Input: part model. Units: mm. Frame: model coordinates. A direction names the side the tool comes from. Give positions to 0.01 mm unless a question says otherwise; leave off trailing zeros. Loops run counter-clockwise (first coordinate to the right, second up) from the corner with the lowest first, then second, coordinate; pieces in that order, holes last. Notation, with made-up numbers: (54.5, 78.5) - (96.5, 78.5) arc R21 cw to (96.5, 106.5) - close; hole circle Ø3 at (69.25, 82.5). An arc over 180 degrees is marked (long way). Answer as a JSON object with one key per item and string values.
from build123d import *

# Parameters (mm, degrees)
BOSS_EXTRUDE1_DEPTH  = 9.2
FILLET1_R            = 0.3
CUT_EXTRUDE1_DEPTH   = 19.2
SKETCH3_W            = 9.9
SKETCH3_H            = 1.3
BOSS_EXTRUDE2_DEPTH  = 6.5
SKETCH4_W            = 0.621842352
SKETCH4_H            = 1.7
CUT_EXTRUDE3_DEPTH   = 16.5
SKETCH5_R            = 1.8
CUT_EXTRUDE4_DEPTH   = 16.5
SKETCH8_W            = 1.27
SKETCH8_H            = 0.5
BOSS_EXTRUDE4_DEPTH  = 1.46
SKETCH9_W            = 1.52
SKETCH9_H            = 0.5
BOSS_EXTRUDE5_DEPTH  = 1
SKETCH10_W           = 1.27
SKETCH10_H           = 0.5
BOSS_EXTRUDE6_DEPTH  = 0.5
SKETCH11_W           = 0.8
SKETCH11_H           = 0.5
BOSS_EXTRUDE7_DEPTH  = 10.08
CHAMFER1_SIZE        = 0.3
CHAMFER2_SIZE        = 0.2
BOSS_EXTRUDE10_DEPTH = 0.05


with BuildPart() as part:
    # Sketch1 → Boss-Extrude1 (new body)
    with BuildSketch(Plane.XY):
        Polygon((1.031077827, 0), (-8.968922173, 0), (-8.575223187, 4.5), (0.637378841, 4.5), align=None)
    extrude(amount=BOSS_EXTRUDE1_DEPTH)

    # Fillet1
    fillet1_edges = [part.edges().sort_by_distance(p)[0] for p in [
        (-8.575223187, 4.5, 4.6),
        (0.637378841, 4.5, 4.6),
    ]]
    fillet(fillet1_edges, radius=FILLET1_R)

    # Sketch2 → Cut-Extrude1 (cut)
    with BuildSketch(Plane(origin=(5, 0, 0), x_dir=(0, 0, -1), z_dir=(1, 0, 0))):
        Polygon((0, 4.5), (-0.279963723, 4.5), (0, 1.3), align=None)
    extrude(amount=-CUT_EXTRUDE1_DEPTH, mode=Mode.SUBTRACT)

    # Sketch3 → Boss-Extrude2 (add)
    with BuildSketch(Plane(origin=(0, 0, 0), x_dir=(-1, 0, 0), z_dir=(0, 0, -1))):
        with Locations((3.968922173, 0.65)):
            Rectangle(SKETCH3_W, SKETCH3_H)
    extrude(amount=BOSS_EXTRUDE2_DEPTH)

    # Sketch4 → Cut-Extrude3 (cut)
    with BuildSketch(Plane(origin=(0, 1.3, 0), x_dir=(1, 0, 0), z_dir=(0, 1, 0))):
        with Locations((-8.608000997, 4.35)):
            Rectangle(SKETCH4_W, SKETCH4_H)
        with Locations((0.670156651, 4.35)):
            Rectangle(SKETCH4_W, SKETCH4_H)
    extrude(amount=-CUT_EXTRUDE3_DEPTH, mode=Mode.SUBTRACT)

    # Sketch5 → Cut-Extrude4 (cut)
    with BuildSketch(Plane(origin=(0, 1.3, 0), x_dir=(1, 0, 0), z_dir=(0, 1, 0))):
        with Locations(Location((-3.968922173, 3.7, 0), (0, 0, 270))):
            Circle(SKETCH5_R)
    extrude(amount=-CUT_EXTRUDE4_DEPTH, mode=Mode.SUBTRACT)

    # Sketch8 → Boss-Extrude4 (add)
    with BuildSketch(Plane.XY.offset(9.2)):
        with Locations((-1.428922173, 2.4)):
            Rectangle(SKETCH8_W, SKETCH8_H)
        with Locations((-3.968922173, 2.4)):
            Rectangle(SKETCH8_W, SKETCH8_H)
        with Locations((-6.508922173, 2.4)):
            Rectangle(SKETCH8_W, SKETCH8_H)
    extrude(amount=BOSS_EXTRUDE4_DEPTH)

    # Sketch9 → Boss-Extrude5 (add)
    with BuildSketch(Plane.XY.offset(10.66)):
        with Locations((-3.968922173, 2.4)):
            Rectangle(SKETCH9_W, SKETCH9_H)
        with Locations((-1.428922173, 2.4)):
            Rectangle(SKETCH9_W, SKETCH9_H)
        with Locations((-6.508922173, 2.4)):
            Rectangle(SKETCH9_W, SKETCH9_H)
    extrude(amount=BOSS_EXTRUDE5_DEPTH)

    # Sketch10 → Boss-Extrude6 (add)
    with BuildSketch(Plane.XY.offset(11.66)):
        with Locations((-3.968922173, 2.4)):
            Rectangle(SKETCH10_W, SKETCH10_H)
        with Locations((-1.428922173, 2.4)):
            Rectangle(SKETCH10_W, SKETCH10_H)
        with Locations((-6.508922173, 2.4)):
            Rectangle(SKETCH10_W, SKETCH10_H)
    extrude(amount=BOSS_EXTRUDE6_DEPTH)

    # Sketch11 → Boss-Extrude7 (add)
    with BuildSketch(Plane.XY.offset(12.16)):
        with Locations((-3.968922173, 2.4)):
            Rectangle(SKETCH11_W, SKETCH11_H)
        with Locations((-1.428922173, 2.4)):
            Rectangle(SKETCH11_W, SKETCH11_H)
        with Locations((-6.508922173, 2.4)):
            Rectangle(SKETCH11_W, SKETCH11_H)
    extrude(amount=BOSS_EXTRUDE7_DEPTH)

    # Chamfer1
    # the kernel refuses this chamfer: 0.3 mm, written as the material it takes off along each edge
    with BuildSketch(Plane(origin=(-0.793922173, 3.421504896, 12.16), x_dir=(-0.9996219169112968, 0, 0.027495876610584464), z_dir=(0, -1, 0))) as chamfer1_piece_1_section:
        Polygon((CHAMFER1_SIZE * 0.999621916911, CHAMFER1_SIZE * 0.0274958766106), (-CHAMFER1_SIZE * 0.0274958766106, CHAMFER1_SIZE * 0.999621916911), (0, 0), align=None)
    chamfer1_piece_1 = extrude(amount=2.043009793, mode=Mode.PRIVATE)
    chamfer1_piece_1 = split(chamfer1_piece_1, bisect_by=Plane(origin=(-1.028922173, 2.4, 12.055687512), z_dir=(1, 0, 0)), keep=Keep.TOP, mode=Mode.PRIVATE)
    add(chamfer1_piece_1, mode=Mode.SUBTRACT)
    with BuildSketch(Plane(origin=(-2.063922173, 1.378495104, 12.16), x_dir=(-0.027495876610585904, 0, -0.9996219169112968), z_dir=(0, 1, 0))) as chamfer1_piece_2_section:
        Polygon((CHAMFER1_SIZE * 0.999621916911, -CHAMFER1_SIZE * 0.0274958766106), (-CHAMFER1_SIZE * 0.0274958766106, -CHAMFER1_SIZE * 0.999621916911), (0, 0), align=None)
    chamfer1_piece_2 = extrude(amount=2.043009793, mode=Mode.PRIVATE)
    chamfer1_piece_2 = split(chamfer1_piece_2, bisect_by=Plane(origin=(-1.828922173, 2.4, 12.055687512), z_dir=(-1, 0, 0)), keep=Keep.TOP, mode=Mode.PRIVATE)
    add(chamfer1_piece_2, mode=Mode.SUBTRACT)
    with BuildSketch(Plane(origin=(-4.603922173, 1.378495104, 12.16), x_dir=(-0.027495876610587344, 0, -0.9996219169112968), z_dir=(0, 1, 0))) as chamfer1_piece_3_section:
        Polygon((CHAMFER1_SIZE * 0.999621916911, -CHAMFER1_SIZE * 0.0274958766106), (-CHAMFER1_SIZE * 0.0274958766106, -CHAMFER1_SIZE * 0.999621916911), (0, 0), align=None)
    chamfer1_piece_3 = extrude(amount=2.043009793, mode=Mode.PRIVATE)
    chamfer1_piece_3 = split(chamfer1_piece_3, bisect_by=Plane(origin=(-4.368922173, 2.4, 12.055687512), z_dir=(-1, 0, 0)), keep=Keep.TOP, mode=Mode.PRIVATE)
    add(chamfer1_piece_3, mode=Mode.SUBTRACT)
    with BuildSketch(Plane(origin=(-3.333922173, 3.421504896, 12.16), x_dir=(-0.9996219169112968, 0, 0.027495876610584506), z_dir=(0, -1, 0))) as chamfer1_piece_4_section:
        Polygon((CHAMFER1_SIZE * 0.999621916911, CHAMFER1_SIZE * 0.0274958766106), (-CHAMFER1_SIZE * 0.0274958766106, CHAMFER1_SIZE * 0.999621916911), (0, 0), align=None)
    chamfer1_piece_4 = extrude(amount=2.043009793, mode=Mode.PRIVATE)
    chamfer1_piece_4 = split(chamfer1_piece_4, bisect_by=Plane(origin=(-3.568922173, 2.4, 12.055687512), z_dir=(1, 0, 0)), keep=Keep.TOP, mode=Mode.PRIVATE)
    add(chamfer1_piece_4, mode=Mode.SUBTRACT)
    with BuildSketch(Plane(origin=(-7.143922173, 1.378495104, 12.16), x_dir=(-0.027495876610587344, 0, -0.9996219169112968), z_dir=(0, 1, 0))) as chamfer1_piece_5_section:
        Polygon((CHAMFER1_SIZE * 0.999621916911, -CHAMFER1_SIZE * 0.0274958766106), (-CHAMFER1_SIZE * 0.0274958766106, -CHAMFER1_SIZE * 0.999621916911), (0, 0), align=None)
    chamfer1_piece_5 = extrude(amount=2.043009793, mode=Mode.PRIVATE)
    chamfer1_piece_5 = split(chamfer1_piece_5, bisect_by=Plane(origin=(-6.908922173, 2.4, 12.055687512), z_dir=(-1, 0, 0)), keep=Keep.TOP, mode=Mode.PRIVATE)
    add(chamfer1_piece_5, mode=Mode.SUBTRACT)
    with BuildSketch(Plane(origin=(-5.873922173, 3.421504896, 12.16), x_dir=(-0.9996219169112968, 0, 0.027495876610584464), z_dir=(0, -1, 0))) as chamfer1_piece_6_section:
        Polygon((CHAMFER1_SIZE * 0.999621916911, CHAMFER1_SIZE * 0.0274958766106), (-CHAMFER1_SIZE * 0.0274958766106, CHAMFER1_SIZE * 0.999621916911), (0, 0), align=None)
    chamfer1_piece_6 = extrude(amount=2.043009793, mode=Mode.PRIVATE)
    chamfer1_piece_6 = split(chamfer1_piece_6, bisect_by=Plane(origin=(-6.108922173, 2.4, 12.055687512), z_dir=(1, 0, 0)), keep=Keep.TOP, mode=Mode.PRIVATE)
    add(chamfer1_piece_6, mode=Mode.SUBTRACT)

    # Chamfer2
    chamfer2_edges = [part.edges().sort_by_distance(p)[0] for p in [
        (-3.568922173, 2.4, 22.24),
        (-4.368922173, 2.4, 22.24),
        (-6.108922173, 2.4, 22.24),
        (-6.908922173, 2.4, 22.24),
        (-1.028922173, 2.4, 22.24),
        (-1.828922173, 2.4, 22.24),
    ]]
    chamfer(chamfer2_edges, length=CHAMFER2_SIZE)

    # Sketch15 → Boss-Extrude10 (add)
    with BuildSketch(Plane(origin=(0, 0, 0), x_dir=(-1, 0, 0), z_dir=(0, -1, 0))):
        Polygon((8.968922173, 0), (7.937844346, 0), (7.937844346, -8.229840369), (0, -8.229840369), (0, 0), (-1.031077827, 0), (-1.031077827, -9.2), (8.968922173, -9.2), align=None)
    extrude(amount=BOSS_EXTRUDE10_DEPTH)


solid = part.part
Item 1: Mould query, pull axis X, two halves, no side actions, for faces 5 (the face through (-8.787, 2.083, 4.536)), 6 (the face through (-4, 0, 1)), 7 (the face through (-4, 1, -6.5)), 8 (the face through (0.981, 1, -2)). Classes: released by +X, released by -X, zero draft, split by the parting line, or undercut.
Geometry check:
{"face 5": "released by -X", "face 6": "undercut", "face 7": "zero draft", "face 8": "released by +X"}
Item 2: Cut plane C-C (z = -1.5). Return loops of the section in (x, y), then the cut area to 3 significant figures.
Geometry check:
{"outline": "(-8.92, 0) - (0.98, 0) - (0.98, 1.3) - (-8.92, 1.3) - close", "area": "12.9 mm2"}
Item 3: Contact query for flat-ended pins moving along their axis: P1, Ø2, axis at y = 3.5, z = 0, coming from the +X side; P2, Ø5, axis at x = -7.5, z = 7, coming from the -Y side; P3, Ø0.6, axis at y = 2.5, z = 10, coming from the -X side; P4, Ø4, axis at x = -5, z = 14.5, coming from the +Y side. Output: stop coordinate, or through.
Geometry check:
{"P1": "stops at x = 0.81", "P2": "stops at y = -0.05", "P3": "stops at x = -7.14", "P4": "stops at y = 2.65"}
Item 4: Cut plane A-A (x = -5.25). Return loops of the section in (y, z), then the cut area to 3 significant figures.
Geometry check:
{"outline": "(-0.05, 8.23) - (0, 8.23) - (0, -2.44) - (1.3, -2.44) - (1.3, 0) - (4.5, 0.28) - (4.5, 9.2) - (-0.05, 9.2) - close; (0, -6.5) - (1.3, -6.5) - (1.3, -4.96) - (0, -4.96) - close", "area": "46.2 mm2"}
Item 5: Material intervals for line 1 (X direction, y = 0.6, z = -3.7); line 2 (Z direction, x = 0.5, y = 0.6); line 3 (Y direction, x = -6, z = 2.5), sorted ascending. Write a range as [from, to].
Geometry check:
{"line 1": "x = [-8.3, -5.77], [-2.17, 0.36]", "line 2": "z = [-6.5, -5.2], [-3.5, 9.2]", "line 3": "y = [0, 4.5]"}
Item 6: Access query for faces 1 (the face through (-3, 1.3, -2)), 2 (the face through (-6.5, 2.15, 15.6)), 3 (the face through (-6.5, 2.65, 15.6)), 4 (the face through (0.359, 1, -4)). Directions: +Z, -Z, +X, -X, +Y, -Y. A direction counts if a zero-diameter tool reaches every point of the face in a straight line with its end or side. Return the directions, or none.
Geometry check:
{"face 1": "-Z, +X, -X, +Y", "face 2": "+Z, +X, -X, -Y", "face 3": "+Z, +X, -X, +Y", "face 4": "+X, +Y, -Y"}
